```python
from build123d import *

# Parameters (mm, degrees)
BASE_EXTRUDE_DEPTH = 3


with BuildPart() as part:
    # Sketch1 → Base-Extrude (new body)
    with BuildSketch(Plane.XY):
        with BuildLine():
            Line((732.034300263, -38.701536799), (738.412696802, -41.20669573))
            Line((738.412696802, -41.20669573), (736.473436897, -43.947731787))
            ThreePointArc((736.473436897, -43.947731787), (735.449310633, -44.697774319), (734.180021911, -44.680323155))
            Line((734.180021911, -44.680323155), (730.013302653, -43.221928834))
            ThreePointArc((730.013302653, -43.221928834), (726.93179591, -40.113817439), (727.477141983, -35.771164112))
            Line((727.477141983, -35.771164112), (731.560851868, -29.509962721))
            ThreePointArc((731.560851868, -29.509962721), (731.992554194, -29.036110484), (732.551993885, -28.723172671))
            Line((732.551993885, -28.723172671), (771.665266629, -14.487105627))
            ThreePointArc((771.665266629, -14.487105627), (776.436585639, -10.825943783), (778.245065196, -5.090179419))
            Line((778.245065196, -5.090179419), (778.245065196, 32.909820581))
            Line((778.245065196, 32.909820581), (787.245065196, 25.583892383))
            Line((787.245065196, 25.583892383), (787.245065196, -7.416107617))
            ThreePointArc((787.245065196, -7.416107617), (786.883369284, -8.563260489), (785.929105482, -9.295492858))
            Line((785.929105482, -9.295492858), (785.06938995, -9.608403722))
            ThreePointArc((785.06938995, -9.608403722), (784.319331429, -10.093744269), (783.855426973, -10.857246649))
            ThreePointArc((783.855426973, -10.857246649), (782.140163623, -14.493920417), (779.609772484, -17.618763634))
            ThreePointArc((779.609772484, -17.618763634), (778.800038242, -18.253560622), (777.875517606, -18.705111674))
            Line((777.875517606, -18.705111674), (744.440455722, -30.874478981))
            ThreePointArc((744.440455722, -30.874478981), (743.317578976, -31.896513164), (743.236121599, -33.412682929))
            Line((743.236121599, -33.412682929), (743.365082604, -33.782324318))
            ThreePointArc((743.365082604, -33.782324318), (743.443954805, -34.801616013), (743.008797081, -35.726718244))
            Line((743.008797081, -35.726718244), (740.445206883, -38.781886072))
            Line((740.445206883, -38.781886072), (733.131014766, -35.909187018))
            Line((733.131014766, -35.909187018), (732.034300263, -38.701536799))
        make_face()
    extrude(amount=BASE_EXTRUDE_DEPTH)


solid = part.part
```
Design review of the part built by this model. Coordinates are the model's own, in mm. A direction names the side the tool comes from. Round coordinates to 2 decimals unless told otherwise and drop trailing zeros. Order: outer loops, then holes, each group sorted by start corner. A loop starts at its lowest first (then second) coordinate and runs counter-clockwise, first axis right, second up. Notation, with made-up numbers: M 23.5,65 L 59.5,65 A30 cw 59.5,104 Z; hole C 19,-27.75 d9. An arc over 180 degrees is marked long. Put each result on its own line as item: value.
Q1. Consider section A-A (z = 1.7). State the section outline as (x, y) points, and give its area (3 significant figures).
Reported:
outline: M 727.48,-35.77 A5 ccw 730.01,-43.22 L 734.18,-44.68 A2 ccw 736.47,-43.95 L 738.41,-41.21 L 732.03,-38.7 L 733.13,-35.91 L 740.45,-38.78 L 743.01,-35.73 A2 ccw 743.37,-33.78 L 743.24,-33.41 A2 cw 744.44,-30.87 L 777.88,-18.71 A4.9 ccw 779.61,-17.62 A16.8 ccw 783.86,-10.86 A2 cw 785.07,-9.61 L 785.93,-9.3 A2 ccw 787.25,-7.42 L 787.25,25.58 L 778.25,32.91 L 778.25,-5.09 A10 cw 771.67,-14.49 L 732.55,-28.72 A2 ccw 731.56,-29.51 Z
area: 812 mm²
Q2. Draft analysis for pull direction Y (two halves, no side actions). For faces 1 (the face through (787.245, 9, 1)), 2 (the face through (743.447, -34.787, 1.479)), 3 (the face through (743.327, -31.877, 1.479)), 4 (the face through (776.387, -10.896, 1.479)), state which applies: released by +Y, released by -Y, zero draft, split by the parting line, or undercut.
Reported:
face 1: zero draft
face 2: undercut
face 3: undercut
face 4: released by +Y
Q3. Consider section B-B (y = -12.5). State the section outline as (x, z) points, and give its area (3 significant figures).
Reported:
outline: M 774.96,0 L 783.21,0 L 783.21,3 L 774.96,3 Z
area: 24.8 mm²
Q4. Consider section C-C (x = 749). State the section outline as (y, z) points, and give its area (3 significant figures).
Reported:
outline: M -29.21,0 L -22.74,0 L -22.74,3 L -29.21,3 Z
area: 19.4 mm²
Q5. Insertion check: pin 1 Ø1.5 at (y, z) = (5.5, 1.5) entering from -X; pin 2 Ø12 at (x, y) = (760, -27) entering from +Z. Each pin has a flat end and moves straight along its axis. Give the tip position at first contact, or say it passes through.
Reported:
pin 1: x = 778.25
pin 2: z = 3
Q6. To check wall thickness, follow line 1 (X direction, y = 12.5, z = 2.55); line 2 (Y direction, x = 736, z = 2.2); line 3 (Y direction, x = 779.5, z = 2.85). State the ranges of each line that lie inside material, in increasing order.
Reported:
line 1: 778.25 to 787.25
line 2: -44.42 to -40.26, -37.04 to -27.47
line 3: -17.72 to 31.89
Q7. Machinability: for faces 5 (the face through (732.126, -43.961, 1.479)), 6 (the face through (778.245, 14, 1)), 7 (the face through (732.59, -37.29, 1.48)), which of the approach directions +Z, -Z, +X, -X, +Y, -Y give a long, thin tool a straight path to every point of the face, cutting with its end or side? Answer none if there is none.
Reported:
face 5: +Z, -Z, -X, -Y
face 6: +Z, -Z, -X, +Y
face 7: +Z, -Z
